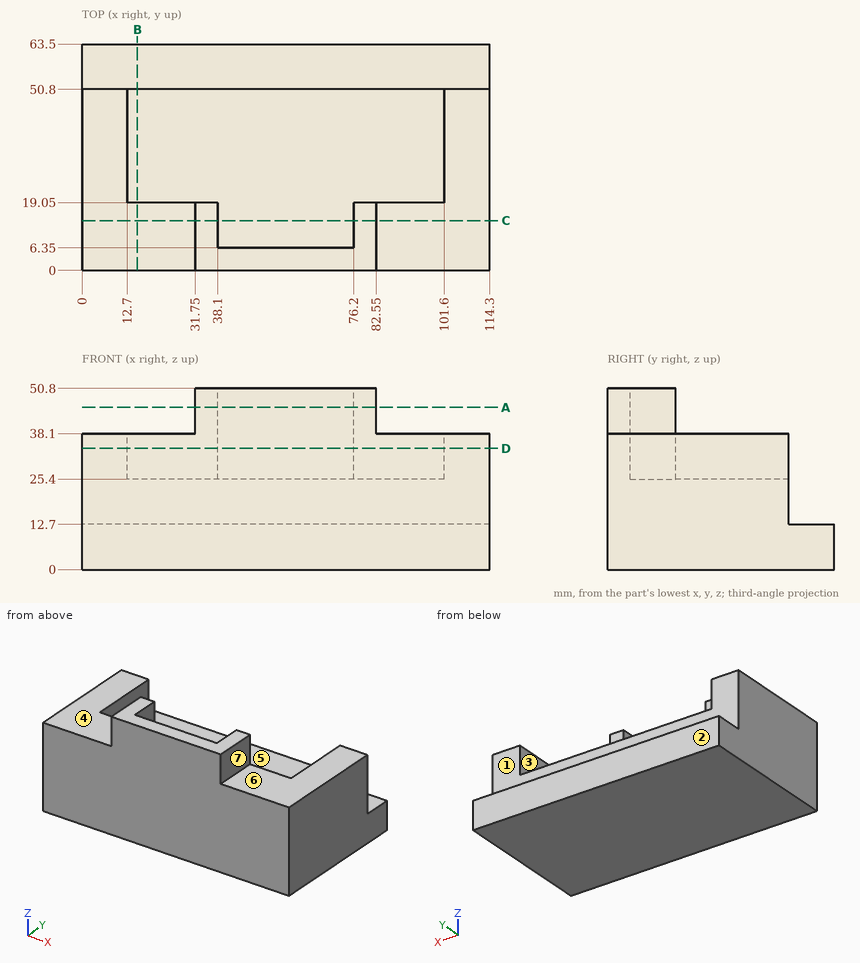
The drawing under review shows one solid part. Ordinate dimensions are in mm from its lowest x, y, z. A direction names the side the tool comes from. Round coordinates to 2 decimals unless told otherwise and drop trailing zeros. Write each loop counter-clockwise with the first axis right and the second up, starting at its lowest first coordinate (ties: lowest second). Pieces come first, ordered by that corner, then holes. Notation, with made-up numbers: M 72.5,40 L 131.5,40 A30 ccw 131.5,70 Z; hole C -33.5,87 d4. An arc over 180 degrees is marked long. One line per item, written item: value. Start each with the question number.
(1) We need section C-C (y = 14). Give the boundary of the cut face in (x, z), and give its area (3 significant figures).
(2) The part is to be moulded in two halves that separate along X. For the marked faces 5, 6 and 7, say which applies: released by +X, released by -X, zero draft, split by the parting line, or undercut.
(3) We need section A-A (z = 45.5). Give the boundary of the cut face in (x, y).
(4) We need section D-D (z = 34). Give the boundary of the cut face in (x, y).
(5) Wall thickness on line 1 (X direction, y = 41, z = 25.5); line 2 (X direction, y = 18, z = 29); line 3 (Z direction, x = 68, y = 14): over which ranges is each line inside the solid? List them lowest first.
(6) Insertion check: pin 1 (16 mm diameter, centred on x = 96.5, y = 20.5, fed in from +Z); pin 2 (20.5 mm diameter, centred on x = 20, z = 40.5, fed in from +Y); pin 3 (12.5 mm diameter, centred on x = 85, z = 37, fed in from +Y). Each pin has a flat end and moves straight along its axis. Give the tip position at first contact, or say it passes through.
(7) We need section B-B (x = 15.5). Give the boundary of the cut face in (y, z), and give its area (3 significant figures).
(8) Machinability: for the marked faces 1, 2, 3 and 4, which of the approach directions +Z, -Z, +X, -X, +Y, -Y give a long, thin tool a straight path to every point of the face, cutting with its end or side? Answer none if there is none.
Result:
1. outline: M 0,0 L 114.3,0 L 114.3,38.1 L 82.55,38.1 L 82.55,50.8 L 76.2,50.8 L 76.2,25.4 L 38.1,25.4 L 38.1,50.8 L 31.75,50.8 L 31.75,38.1 L 0,38.1 Z
1. area: 4,030 mm²
2. face 5: undercut
2. face 6: zero draft
2. face 7: released by +X
3. outline: M 31.75,0 L 82.55,0 L 82.55,19.05 L 76.2,19.05 L 76.2,6.35 L 38.1,6.35 L 38.1,19.05 L 31.75,19.05 Z
4. outline: M 0,0 L 114.3,0 L 114.3,50.8 L 101.6,50.8 L 101.6,19.05 L 76.2,19.05 L 76.2,6.35 L 38.1,6.35 L 38.1,19.05 L 12.7,19.05 L 12.7,50.8 L 0,50.8 Z
5. line 1: 0 to 12.7, 101.6 to 114.3
5. line 2: 0 to 38.1, 76.2 to 114.3
5. line 3: 0 to 25.4
6. pin 1: z = 38.1
6. pin 2: y = 50.8
6. pin 3: y = 19.05
7. outline: M 0,0 L 63.5,0 L 63.5,12.7 L 50.8,12.7 L 50.8,25.4 L 19.05,25.4 L 19.05,38.1 L 0,38.1 Z
7. area: 1,690 mm²
8. face 1: +Z, +X, -X, +Y
8. face 2: +Z, -Z, +X, -X, +Y
8. face 3: +Z, +Y
8. face 4: +Z, -X, +Y, -Y
